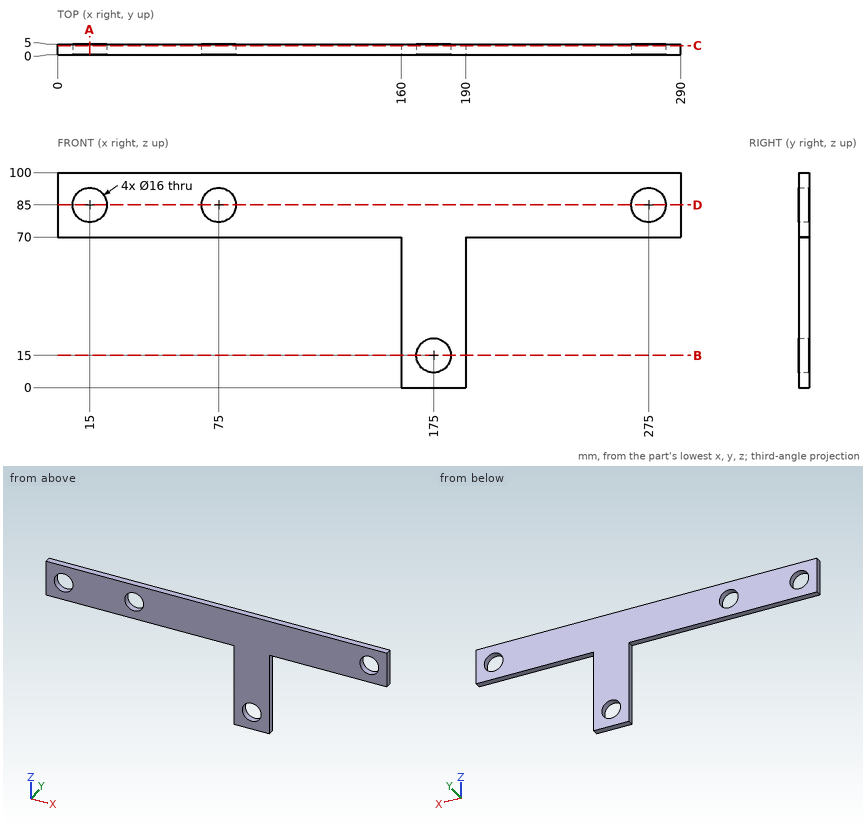
Source: three-view drawing plus pictorial views. Frame: mm from the lowest corner of the part. Give positions to 0.01 mm unless a question says otherwise; leave off trailing zeros. Loops run counter-clockwise (first coordinate to the right, second up) from the corner with the lowest first, then second, coordinate; pieces in that order, holes last. Notation, with made-up numbers: (66.5, -13.5) -> (83.5, -13.5) arc R17 ccw to (83.5, 8.5) -> close; hole circle Ø3 at (18, 27.5). An arc over 180 degrees is marked (long way). Use a Markdown table: item, result. Add a question column.
(1) First-contact query: pin 1 Ø1.5 at (x, y) = (40.5, 2) entering from -Z; pin 2 Ø1.5 at (y, z) = (3.5, 48) entering from -X; pin 3 Ø3 at (y, z) = (1.5, 43) entering from +X. Flat tips, straight axial feed; report the tip coordinate or a pass-through.
(2) Section query B-B (z = 15). Output: boundary loops of the cut face in (x, y).
(3) Ray query, line 1 (X direction, y = 1.4, z = 85); line 2 (X direction, y = 2.5, z = 15); line 3 (Z direction, x = 275, y = 2.8). Return the intervals inside material, ascending.
(4) Section query C-C (y = 4.2). Output: boundary loops of the cut face in (x, z), then the cut area to 4 significant figures.
(5) Section query A-A (x = 15). Output: boundary loops of the cut face in (y, z).
(6) Section query D-D (z = 85). Output: boundary loops of the cut face in (x, y).
Checked values:
| question | item | result |
|---|---|---|
| 1 | pin 1 | z = 70 |
| 1 | pin 2 | x = 160 |
| 1 | pin 3 | x = 190 |
| 2 | outline | (160, 0) -> (167, 0) -> (167, 5) -> (160, 5) -> close; (183, 0) -> (190, 0) -> (190, 5) -> (183, 5) -> close |
| 3 | line 1 | 0 to 7, 23 to 67, 83 to 267, 283 to 290 |
| 3 | line 2 | 160 to 167, 183 to 190 |
| 3 | line 3 | 70 to 77, 93 to 100 |
| 4 | outline | (0, 70) -> (160, 70) -> (160, 0) -> (190, 0) -> (190, 70) -> (290, 70) -> (290, 100) -> (0, 100) -> close; hole circle Ø16 at (15, 85); hole circle Ø16 at (75, 85); hole circle Ø16 at (175, 15); hole circle Ø16 at (275, 85) |
| 4 | area | 10,000 mm^2 |
| 5 | outline | (0, 70) -> (5, 70) -> (5, 77) -> (0, 77) -> close; (0, 93) -> (5, 93) -> (5, 100) -> (0, 100) -> close |
| 6 | outline | (0, 0) -> (7, 0) -> (7, 5) -> (0, 5) -> close; (23, 0) -> (67, 0) -> (67, 5) -> (23, 5) -> close; (83, 0) -> (267, 0) -> (267, 5) -> (83, 5) -> close; (283, 0) -> (290, 0) -> (290, 5) -> (283, 5) -> close |
